```python
from build123d import *

# Parameters (mm, degrees)
F0_R     = 4
F1_DEPTH = 1
F2_R     = 3
F3_DEPTH = 6
F6_W     = 2
F6_H     = 8.928134
F6_W_2   = 2.979646
F7_DEPTH = 12.5
F8_R     = 1
F9_DEPTH = 6.001


with BuildPart() as f1:
    # F0 (on Top) → F1 (new body)
    with BuildSketch(Plane.XY):
        Circle(F0_R)
    extrude(amount=F1_DEPTH)

    # F2 (on face) → F3 (join)
    with BuildSketch(Plane.XY.offset(1)):
        Circle(F2_R)
    extrude(amount=F3_DEPTH)

    # F4 (on face) → F5 (revolve)
    with BuildSketch(Plane.XY.offset(7)):
        with BuildLine():
            ThreePointArc((0, -3), (2.12132, -2.12132), (3, 0))
            ThreePointArc((3, 0), (2.12132, 2.12132), (0, 3))
            Line((0, 3), (0, -3))
        make_face()
    revolve(axis=Axis((0, 0, 7), (0, -1, 0)))

    # F6 (on Front) → F7 (cut, symmetric)
    with BuildSketch(Plane.XZ):
        with Locations((0, 7.464067)):
            Rectangle(F6_W, F6_H)
        with Locations((-3.489823, 7.464067)):
            Rectangle(F6_W_2, F6_H)
        with Locations((3.489823, 7.464067)):
            Rectangle(F6_W_2, F6_H)
    extrude(amount=F7_DEPTH, both=True, mode=Mode.SUBTRACT)

    # F8 (on face) → F9 (cut, through all)
    with BuildSketch(Plane(origin=(-2, 0, 0), x_dir=(0, -1, 0), z_dir=(-1, 0, 0))):
        with Locations((0, 6.470004)):
            Circle(F8_R)
    extrude(amount=-F9_DEPTH, mode=Mode.SUBTRACT)


solid = f1.part
```
Geometry check sheet. Reference: the model listing, model coordinates, mm. A direction names the side the tool comes from. Coordinates: 2 decimals unless noted, no trailing zeros. Order: outer loops, then holes, each group sorted by start corner. A loop starts at its lowest first (then second) coordinate and runs counter-clockwise, first axis right, second up. Notation, with made-up numbers: (-31, -37) - (-6, -37) arc R18 cw to (-6, -25) - close; hole circle Ø2 at (7.5, -1.5). An arc over 180 degrees is marked (long way). Answer in a Markdown table with one row per item. Add a question column.
1. Draft check along Y on faces 1 (the face through (-0.867, -3.905, 0.493)), 2 (the face through (1.49, 0.13, 7.46)), 3 (the face through (1, 0, 5)). Enter one of: +Y half, -Y half, draft (parallel to the pull), parting line (faces both ways), or undercut.
2. Material ranges on L1, parallel to X at y = 1.25, z = 4.5; L2, parallel to Z at x = 0.5, y = -3.5; L3, parallel to Z at x = 1.3, y = 0, recorded low to high. Write a range as [from, to].
3. Section check C-C (z = 1.5). Enter the section's corners in (x, y).
4. Access from +Z, -Z, +X, -X, +Y, -Y to the whole of each face (thin tool, end or side, straight path). Record for faces 4 (the face through (1, 3, 1)), 5 (the face through (2.4, 0, 3)), 6 (the face through (-2.4, 0, 3)), 7 (the face through (0, 0, 3)).
5. Section check B-B (x = 0). Enter the section's corners in (y, z), plus the area to 3 significant figures.
6. Section check A-A (z = 5.25). Enter the section's corners in (x, y).
7. Gauge pin test, flat ends, axial feed: pin 1 Ø3 at (y, z) = (0, 6.47) entering from +X; pin 2 Ø1 at (x, y) = (-3, 3) entering from +Z; pin 3 Ø3 at (y, z) = (1, 5) entering from -X; pin 4 Ø1 at (x, y) = (2, 1) entering from -Z. Record the tip position at first contact, or that the pin passes through.
Data:
| question | item | result |
|---|---|---|
| 1 | face 1 | parting line |
| 1 | face 2 | undercut |
| 1 | face 3 | draft |
| 2 | L1 | x = [-2, -1], [1, 2] |
| 2 | L2 | z = [0, 1] |
| 2 | L3 | z = [0, 5.47], [7.47, 9.7] |
| 3 | outline | circle Ø6 at (0, 0) |
| 4 | face 4 | +Z |
| 4 | face 5 | +Z, +X, +Y, -Y |
| 4 | face 6 | +Z, -X, +Y, -Y |
| 4 | face 7 | +Z, +Y, -Y |
| 5 | outline | (-4, 0) - (4, 0) - (4, 1) - (3, 1) - (3, 3) - (-3, 3) - (-3, 1) - (-4, 1) - close |
| 5 | area | 20.0 mm² |
| 6 | outline | (-2, -2.24) arc R3 ccw to (-1, -2.83) - (-1, 2.83) arc R3 ccw to (-2, 2.24) - close; (1, -2.83) arc R3 ccw to (2, -2.24) - (2, 2.24) arc R3 ccw to (1, 2.83) - close |
| 7 | pin 1 | stops at x = 2 |
| 7 | pin 2 | stops at z = 1 |
| 7 | pin 3 | stops at x = -2 |
| 7 | pin 4 | stops at z = 0 |
